Read the model definition and answer for the solid it produces. Units are mm, in the model's axes. A direction names the side the tool comes from. Coordinates: 2 decimals unless noted, no trailing zeros. Loops run counter-clockwise (first coordinate to the right, second up) from the corner with the lowest first, then second, coordinate; pieces in that order, holes last. Notation, with made-up numbers: (11.25, 65) -> (62.25, 65) arc R29 ccw to (62.25, 102) -> close; hole circle Ø1 at (38.5, 40.5). An arc over 180 degrees is marked (long way). Answer as a JSON object with one key per item and string values. Group by question number.
Q1. The part is cut by section C-C on x = 205.5. Write down the section's boundary in (y, z), and give its area (3 significant figures).
Q2. Each of these flat-tipped pins is pushed along its axis until it touches: P1, Ø11.5, axis at x = 200.5, y = 18, coming from the -Z side; P2, Ø2, axis at y = 77, z = -14, coming from the -X side; P3, Ø15, axis at x = 63.5, z = -26, coming from the +Y side. Where does it stop, or does it pass through?
Q3. Straight lines are drawn through the part: line 1 along Y through (x, z) = (258, -12.5); line 2 along Z through (x, y) = (312.5, 5); line 3 along Z through (x, y) = (139.5, 33). For each, find the intervals that lie inside material, in ascending order. Write a range as [from, to].
Q4. The part is cut by section B-B on y = 81. Write down the section's boundary in (x, z).
Q5. For faces 1 (the flat face through (126, 19, 0)), 2 (the cylindrical face through (-80.12, 63.14, -16.58)), determine the directions among +Z, -Z, +X, -X, +Y, -Y from which every point of the face is accessible in a straight line to the end or side of a thin tool.
Q6. The part is cut by section A-A on x = -54. Write down the section's boundary in (y, z), and give its area (3 significant figures).
from build123d import *

# Parameters (mm, degrees)
SALIENTE_EXTRUIR1_DEPTH = 38.1
CORTAR_EXTRUIR18_DEPTH  = 38.1
CROQUIS5_R              = 19.05
SALIENTE_EXTRUIR2_DEPTH = 50.8


with BuildPart() as part:
    # Croquis1 → Saliente-Extruir1 (new body)
    with BuildSketch(Plane(origin=(0, 0, 0), x_dir=(1, 0, 0), z_dir=(0, 1, 0))):
        with BuildLine():
            Line((-61.958802083, 0), (319.041197917, 0))
            ThreePointArc((319.041197917, 0), (343.15003125, 26.627666667), (316.522364583, 50.7365))
            Line((316.522364583, 50.7365), (-64.477635417, 50.7365))
            ThreePointArc((-64.477635417, 50.7365), (-88.58646875, 24.108833333), (-61.958802083, 0))
        make_face()
    extrude(amount=SALIENTE_EXTRUIR1_DEPTH)

    # Croquis3 → Cortar-Extruir18 (cut)
    with BuildSketch(Plane(origin=(0, 38.1, 0), x_dir=(1, 0, 0), z_dir=(0, 1, 0))):
        with BuildLine():
            add(Edge.make_bspline(
                [(68.053382641, 25.36825), (85.128897701, 37.242607365), (117.715779547, 53.529246636), (147.710358419, 35.418129568), (159.94527156, 27.422727745)],
                knots=[0.293668056, 0.293668056, 0.293668056, 0.293668056, 0.509999468, 0.663692502, 0.663692502, 0.663692502, 0.663692502], degree=3))
            add(Edge.make_bspline(
                [(68.053382641, 25.36825), (85.297187869, 13.221681932), (118.362782549, -4.355831371), (146.208725565, 18.171330049), (158.923925731, 26.746070777), (159.94527156, 27.422727745)],
                knots=[0.293535528, 0.293535528, 0.293535528, 0.293535528, 0.509769313, 0.658147643, 0.671041491, 0.671041491, 0.671041491, 0.671041491], degree=3))
        make_face()
    extrude(amount=-CORTAR_EXTRUIR18_DEPTH, mode=Mode.SUBTRACT)

    # Croquis5 → Saliente-Extruir2 (add)
    with BuildSketch(Plane(origin=(0, 38.1, 0), x_dir=(1, 0, 0), z_dir=(0, 1, 0))):
        with Locations(Location((-63.21821875, 25.36825, 0), (0, 0, 270))):
            Circle(CROQUIS5_R)
    extrude(amount=SALIENTE_EXTRUIR2_DEPTH)


solid = part.part
Final values:
{
 "1": {"outline": "(0, -50.74) -> (38.1, -50.74) -> (38.1, 0) -> (0, 0) -> close", "area": "1,930 mm2"},
 "2": {"P1": "stops at z = -50.74", "P2": "stops at x = -79.2", "P3": "stops at y = 38.1"},
 "3": {"line 1": "y = [0, 38.1]", "line 2": "z = [-50.74, 0]", "line 3": "z = [-50.74, -39.29], [-13.53, 0]"},
 "4": {"outline": "circle Ø38.1 at (-63.22, -25.37)"},
 "5": {"face 1": "+Z, +X, -X, +Y, -Y", "face 2": "+Y"},
 "6": {"outline": "(0, -50.74) -> (38.1, -50.74) -> (38.1, -42.04) -> (88.9, -42.04) -> (88.9, -8.7) -> (38.1, -8.7) -> (38.1, 0) -> (0, 0) -> close", "area": "3,630 mm2"}
}
